Study the drawing (mm; zero at the part's minimum x, y, z) and answer. A direction names the side the tool comes from. Give positions to 0.01 mm unless a question says otherwise; leave off trailing zeros. Loops run counter-clockwise (first coordinate to the right, second up) from the corner with the lowest first, then second, coordinate; pieces in that order, holes last. Notation, with made-up numbers: M 69.5,83.25 L 106.5,83.25 A18 cw 106.5,104.25 Z; hole C 58,-37.5 d7. An arc over 180 degrees is marked long. Use one line per item in the form item = value. Start each with the question number.
1. The part is cut by section A-A (x = 12.5). Write down the section's boundary in (y, z), and give its area (3 significant figures).
2. The part is cut by section C-C (y = 24.5). Write down the section's boundary in (x, z).
3. Each of these flat-tipped pins is pushed along its axis until it touches: pin 1 Ø10 at (x, z) = (6.5, 18.5) entering from -Y; pin 2 Ø1.5 at (x, y) = (16.5, 5) entering from +Z; pin 3 Ø6 at (x, y) = (9, 7) entering from -Z; pin 4 Ø1 at (x, y) = (3, 18) entering from -Z. Where does it stop, or does it pass through?
4. The part is cut by section B-B (z = 12.5). Write down the section's boundary in (x, y).
5. Straight lines are drawn through the part: line 1 (Y direction, x = 7.75, z = 23); line 2 (Z direction, x = 12.5, y = 6.75); line 3 (X direction, y = 7.75, z = 9.25). For each, find the intervals that lie inside material, in ascending order. Write a range as from..to.
6. For the marked faces 4 and 5, determine the directions among +Z, -Z, +X, -X, +Y, -Y from which every point of the face is accessible in a straight line to the end or side of a thin tool.
7. The part is cut by section D-D (x = 6.25). Write down the section's boundary in (y, z).
8. The mould has two halves that part along Z. Classify the marked faces 1, 2 and 3: released by +Z, released by -Z, zero draft, split by the parting line, or undercut.
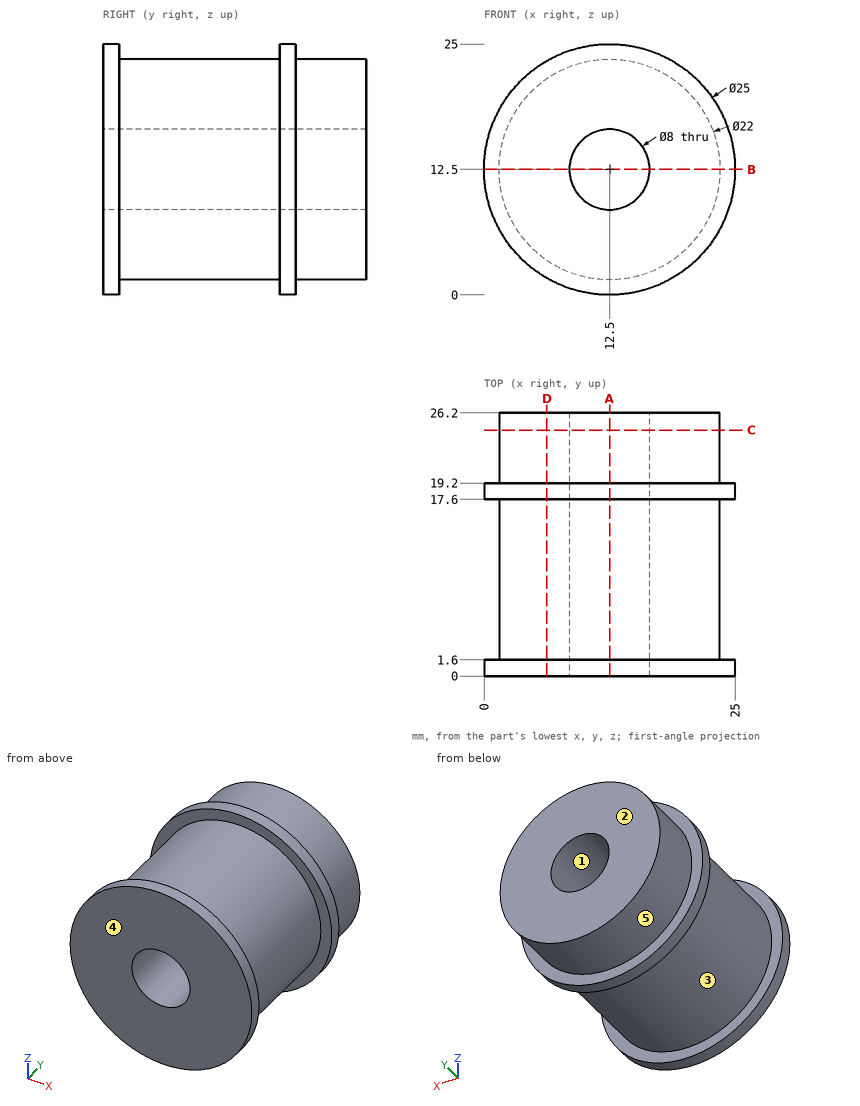
Derived:
q1.outline = M 0,0 L 1.6,0 L 1.6,1.5 L 17.6,1.5 L 17.6,0 L 19.2,0 L 19.2,1.5 L 26.2,1.5 L 26.2,8.5 L 0,8.5 Z; M 0,16.5 L 26.2,16.5 L 26.2,23.5 L 19.2,23.5 L 19.2,25 L 17.6,25 L 17.6,23.5 L 1.6,23.5 L 1.6,25 L 0,25 Z
q1.area = 376 mm2
q2.outline = C 12.5,12.5 d22; hole C 12.5,12.5 d8
q3.pin_1 = 0
q3.pin_2 = 23.01
q3.pin_3 = 1.51
q3.pin_4 = 3.83
q4.outline = M 0,0 L 8.5,0 L 8.5,26.2 L 1.5,26.2 L 1.5,19.2 L 0,19.2 L 0,17.6 L 1.5,17.6 L 1.5,1.6 L 0,1.6 Z; M 16.5,0 L 25,0 L 25,1.6 L 23.5,1.6 L 23.5,17.6 L 25,17.6 L 25,19.2 L 23.5,19.2 L 23.5,26.2 L 16.5,26.2 Z
q5.line_1 = 0..1.6, 17.6..19.2
q5.line_2 = 1.5..8.5, 16.5..23.5
q5.line_3 = 1.99..10.17, 14.83..23.01
q6.face_4 = +Z, -Z, +X, -X, -Y
q6.face_5 = +Y
q7.outline = M 0,1.67 L 1.6,1.67 L 1.6,3.45 L 17.6,3.45 L 17.6,1.67 L 19.2,1.67 L 19.2,3.45 L 26.2,3.45 L 26.2,21.55 L 19.2,21.55 L 19.2,23.33 L 17.6,23.33 L 17.6,21.55 L 1.6,21.55 L 1.6,23.33 L 0,23.33 Z
q8.face_1 = undercut
q8.face_2 = zero draft
q8.face_3 = split by the parting line
